Part model, mm, in its own coordinate system. A direction names the side the tool comes from. Give positions to 0.01 mm unless a question says otherwise; leave off trailing zeros. Write each loop counter-clockwise with the first axis right and the second up, starting at its lowest first coordinate (ties: lowest second). Pieces come first, ordered by that corner, then holes. Notation, with made-up numbers: M -31,24.5 L 7,24.5 A28 ccw 7,57.5 Z; hole C 86.25,84.5 d1. An arc over 180 degrees is marked long. Write item = value, one per line. Start each with the question number.
from build123d import *

# Parameters (mm, degrees)
SKETCH1_R                  = 70
BOSS_EXTRUDE1_DEPTH        = 10
SKETCH2_R                  = 2.65
WYTNIJ_WYCI_GNI_CIE1_DEPTH = 10
SZKIC1_R                   = 5
WYTNIJ_WYCI_GNI_CIE2_DEPTH = 2
SZYK_KO_OWY1_COUNT         = 4
SFAZOWANIE1_SIZE           = 2


with BuildPart() as part:
    # Sketch1 → Boss-Extrude1 (new body)
    with BuildSketch(Plane.XY):
        with BuildLine():
            Line((84.976467331, -2), (77.499555144, -2))
            Line((77.499555144, -2), (77.499555144, 2))
            Line((77.499555144, 2), (84.976467331, 2))
            ThreePointArc((84.976467331, 2), (60.104076401, 60.104076401), (2, 84.976467331))
            Line((2, 84.976467331), (2, 77.499555144))
            Line((2, 77.499555144), (-2, 77.499555144))
            Line((-2, 77.499555144), (-2, 84.976467331))
            ThreePointArc((-2, 84.976467331), (-60.104076401, 60.104076401), (-84.976467331, 2))
            Line((-84.976467331, 2), (-77.499555144, 2))
            Line((-77.499555144, 2), (-77.499555144, -2))
            Line((-77.499555144, -2), (-84.976467331, -2))
            ThreePointArc((-84.976467331, -2), (-60.104076401, -60.104076401), (-2, -84.976467331))
            Line((-2, -84.976467331), (-2, -77.499555144))
            Line((-2, -77.499555144), (2, -77.499555144))
            Line((2, -77.499555144), (2, -84.976467331))
            ThreePointArc((2, -84.976467331), (60.104076401, -60.104076401), (84.976467331, -2))
        make_face()
        Circle(SKETCH1_R, mode=Mode.SUBTRACT)
    extrude(amount=BOSS_EXTRUDE1_DEPTH)

    # Sketch2 → Wytnij-wyciągnięcie1 (cut)
    with BuildSketch(Plane(origin=(0, 0, 0), x_dir=(-1, 0, 0), z_dir=(0, 0, -1))):
        with Locations((-54.800775542, 54.800775542)):
            Circle(SKETCH2_R)
        with Locations((54.800775542, 54.800775542)):
            Circle(SKETCH2_R)
        with Locations((54.800775542, -54.800775542)):
            Circle(SKETCH2_R)
        with Locations((-54.800775542, -54.800775542)):
            Circle(SKETCH2_R)
    extrude(amount=-WYTNIJ_WYCI_GNI_CIE1_DEPTH, mode=Mode.SUBTRACT)

    # Szkic1 → Wytnij-wyciągnięcie2 (cut)
    with BuildSketch(Plane(origin=(0, 0, 0), x_dir=(-1, 0, 0), z_dir=(0, 0, -1))):
        with Locations((-54.800775542, 54.800775542)):
            Circle(SZKIC1_R)
    wytnij_wyci_gni_cie2 = extrude(amount=-WYTNIJ_WYCI_GNI_CIE2_DEPTH, mode=Mode.SUBTRACT)

    # Szyk kołowy1: Wytnij-wyciągnięcie2 ×4 about axis
    szyk_ko_owy1_axis = Axis((0, 0, 0), (0, 0, 1))
    for i in range(1, SZYK_KO_OWY1_COUNT):
        add(wytnij_wyci_gni_cie2.rotate(szyk_ko_owy1_axis, i * 360 / SZYK_KO_OWY1_COUNT), mode=Mode.SUBTRACT)

    # Sfazowanie1
    sfazowanie1_edges = [part.edges().sort_by_distance(p)[0] for p in [
        (57.450775542, -54.800775542, 10),
        (-52.150775542, -54.800775542, 10),
        (-52.150775542, 54.800775542, 10),
        (57.450775542, 54.800775542, 10),
    ]]
    chamfer(sfazowanie1_edges, length=SFAZOWANIE1_SIZE)


solid = part.part
Q1. Drop flat-ended pins along their axis: P1, Ø2, axis at y = 79.5, z = 3, coming from the -X side; P2, Ø8.5, axis at x = -54.8, y = -54.8, coming from the +Z side; P3, Ø6, axis at y = -40, z = 6.5, coming from the +X side; P4, Ø5, axis at x = 54.8, y = -54.8, coming from the +Z side. Give the stop position or say it passes through.
Q2. Slice it at A-A (y = 0). Give the cut face in (x, z).
Q3. Two-plate mould, pull along X, no slides. Class faces 1 (the face through (55.146, -52.173, 4.958)), 2 (the face through (-52.6, 52.6, 2)), 3 (the face through (60.7, 59.5, 4.9)), 4 (the face through (-32, -63, 0)): +X half, -X half, draft (parallel to the pull), parting line (faces both ways), or undercut.
Q4. Probe line 1 along Y through (x, z) = (56, 8); line 2 along X through (y, z) = (57, 8.5); line 3 along Y through (x, z) = (-58, 0.5). List the from-to ranges inside material, lowest first.
Q5. Tool access for faces 5 (the face through (81, -2, 5)), 6 (the face through (0, 77.5, 5)), 7 (the face through (49.92, -55.88, 0.99)): list every direction of +Z, -Z, +X, -X, +Y, -Y with a clear straight run to the whole face (end or side of a thin tool).
Q6. Slice it at C-C (z = 6.5). Give the cut face in (x, y), and give its area (3 significant figures).
Q7. Slice it at D-D (y = 73). Give the cut face in (x, z).
Working result:
q1.P1 = -32.6
q1.P2 = 9.6
q1.P3 = 76.52
q1.P4 = through
q2.outline = M -77.5,0 L -70,0 L -70,10 L -77.5,10 Z; M 70,0 L 77.5,0 L 77.5,10 L 70,10 Z
q3.face_1 = undercut
q3.face_2 = undercut
q3.face_3 = +X half
q3.face_4 = draft
q4.line_1 = -63.95 to -57.16, -52.44 to -42, 42 to 52.44, 57.16 to 63.95
q4.line_2 = -63.06 to -57.06, -52.55 to -40.63, 40.63 to 52.55, 57.06 to 63.06
q4.line_3 = -62.14 to -58.64, -50.96 to -39.19, 39.19 to 50.96, 58.64 to 62.14
q5.face_5 = +Z, -Z, +X
q5.face_6 = +Z, -Z, +Y
q5.face_7 = -Z
q6.outline = M -84.98,-2 A85 ccw -2,-84.98 L -2,-77.5 L 2,-77.5 L 2,-84.98 A85 ccw 84.98,-2 L 77.5,-2 L 77.5,2 L 84.98,2 A85 ccw 2,84.98 L 2,77.5 L -2,77.5 L -2,84.98 A85 ccw -84.98,2 L -77.5,2 L -77.5,-2 Z; hole C 0,0 d140; hole C -54.8,-54.8 d5.3; hole C -54.8,54.8 d5.3; hole C 54.8,-54.8 d5.3; hole C 54.8,54.8 d5.3
q6.area = 7,100 mm2
q7.outline = M -43.54,0 L 43.54,0 L 43.54,10 L -43.54,10 Z
